Geometry: final body of the model. Coordinates: model frame, mm. Face numbers are marked on the shaded views. A direction names the side the tool comes from. Give positions to 0.01 mm unless a question says otherwise; leave off trailing zeros. Order: outer loops, then holes, each group sorted by start corner. A loop starts at its lowest first (then second) coordinate and runs counter-clockwise, first axis right, second up. Notation, with made-up numbers: (69.5, -38.75) - (107.5, -38.75) arc R23 cw to (107.5, 0.25) - close; hole circle Ø11 at (-10.5, 61.5). An arc over 180 degrees is marked (long way). Put each result on its own line as item: value. Start each with the question number.
1. Set-up query: the marked faces 4, 5, 6 and 7. Return all of +Z, -Z, +X, -X, +Y, -Y with unobstructed straight access to the full face (end or side cutting, diameter ignored); none if empty.
2. First-contact query: P1, Ø0.9, axis at x = 3, z = -3.5, coming from the +Y side; P2, Ø3.5, axis at x = -2, z = 17, coming from the -Y side; P3, Ø1, axis at x = 7, z = -1, coming from the +Y side. Flat tips, straight axial feed; report the tip coordinate or a pass-through.
3. Mould query, pull axis Z, two halves, no side actions, for the marked faces 1, 2 and 3. Classes: pulls with the +Z half, pulls with the -Z half, needs draft (parallel to the pull), parting line crosses it, or undercut.
4. Ray query, line 1 along Z through (x, y) = (-5.75, -13); line 2 along Z through (x, y) = (7.75, -20.5); line 3 along Z through (x, y) = (10.75, -16.5). Return the intervals inside material, ascending. Write a range as from..to.
5. Section B-B on x = 6.5. Count the separate pieces of the cut face and the enclosed holes in it, plus the area to 3 significant figures.
6. Section A-A on z = 17.5. Return the cut outline in (x, y).
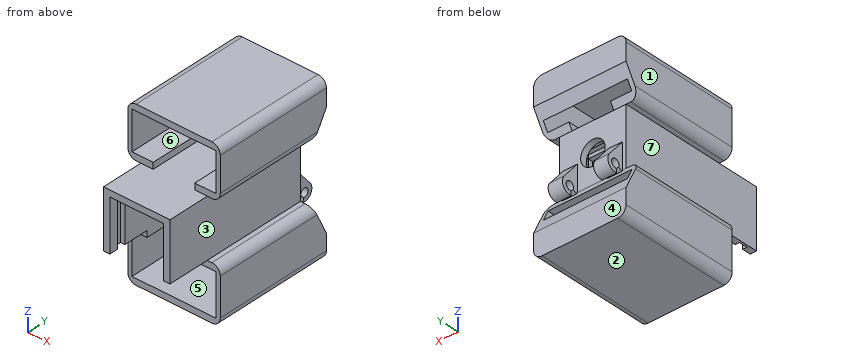
from build123d import *

# Parameters (mm, degrees)
SKETCH_1_W               = 12.8
SKETCH_1_H               = 10.8
EXTRUDE_1_DEPTH          = 1.5
CUT_EXTRUDE_1_REACH      = 13.721
SKETCH_2_R               = 2.9
SKETCH_3_W               = 12.8
SKETCH_3_H               = 1.5
EXTRUDE_2_DEPTH          = 35
SKETCH_6_W               = 12.8
SKETCH_6_H               = 1.5
CUT_EXTRUDE_2_DEPTH      = 10
EXTRUDE_4_DEPTH          = 15.8
CUT_EXTRUDE_3_DEPTH      = 38.580939349
CUT_EXTRUDE_3_DEPTH_BACK = 38.580939349
SKETCH_10_W              = 7.4
SKETCH_10_H              = 4
SKETCH_10_W_2            = 0.8
EXTRUDE_5_DEPTH          = 3.1
EXTRUDE_5_DEPTH_BACK     = 18.9
SKETCH_18_W              = 20
SKETCH_18_H              = 10
CUT_EXTRUDE_4_DEPTH      = 27
CUT_EXTRUDE_5_REACH      = 40.777
SKETCH_20_W              = 12.8
SKETCH_20_H              = 11.75
FILLET_3_R               = 2
SKETCH_21_W              = 12.8
SKETCH_21_H              = 33.5
EXTRUDE_6_DEPTH          = 0.8
SKETCH_22_W              = 12.8
SKETCH_22_H              = 10
CUT_EXTRUDE_6_DEPTH      = 0.8
SKETCH_23_W              = 12.8
SKETCH_23_H              = 2
CUT_EXTRUDE_7_DEPTH      = 0.8
SKETCH_25_W              = 12.8
SKETCH_25_H              = 2
CUT_EXTRUDE_8_DEPTH      = 0.8
SKETCH_26_W              = 12.8
SKETCH_26_H              = 2
CUT_EXTRUDE_9_DEPTH      = 0.8
SKETCH_27_W              = 12.8
SKETCH_27_H              = 2
CUT_EXTRUDE_10_DEPTH     = 0.8
SKETCH_28_W              = 10
SKETCH_28_H              = 2
CUT_EXTRUDE_11_DEPTH     = 0.3
SKETCH_29_W              = 10
SKETCH_29_H              = 2
CUT_EXTRUDE_12_DEPTH     = 0.3
SKETCH_30_W              = 22
SKETCH_30_H              = 28.5
EXTRUDE_7_DEPTH          = 12.2
SKETCH_32_W              = 20
SKETCH_32_H              = 9.2
CUT_EXTRUDE_13_DEPTH     = 27
CUT_EXTRUDE_14_DEPTH     = 46.551260858
SKETCH_34_W              = 9.9
SKETCH_34_H              = 1.5
CUT_EXTRUDE_15_DEPTH     = 39.481186787
FILLET_4_R               = 2
SKETCH_36_W              = 12.3
SKETCH_36_H              = 2
CUT_EXTRUDE_18_DEPTH     = 1
SKETCH_37_W              = 12.3
SKETCH_37_H              = 2
CUT_EXTRUDE_19_DEPTH     = 1


with BuildPart() as part:
    # 草图1 → 凸台-拉伸1 (new body)
    with BuildSketch(Plane(origin=(0, 0, 0), x_dir=(1, 0, 0), z_dir=(0, 1, 0))):
        with Locations((2.081833616, -2.548726655)):
            Rectangle(SKETCH_1_W, SKETCH_1_H)
    extrude(amount=EXTRUDE_1_DEPTH)

    # 草图2 → 切除-拉伸1 (cut, up to next)
    with BuildSketch(Plane(origin=(0, 1.5, 0), x_dir=(1, 0, 0), z_dir=(0, 1, 0)), mode=Mode.PRIVATE) as cut_extrude_1_sk1:
        with Locations(Location((2.081833616, -2.548726655, 0), (0, 0, 270))):
            Circle(SKETCH_2_R)
    cut_extrude_1_tool1 = extrude(cut_extrude_1_sk1.sketch, amount=-CUT_EXTRUDE_1_REACH, mode=Mode.PRIVATE) & part.part
    add(cut_extrude_1_tool1.solids().sort_by_distance((2.081834, 1.5, 2.548727))[0], mode=Mode.SUBTRACT)

    # 草图3 → 凸台-拉伸2 (add)
    with BuildSketch(Plane(origin=(0, 1.5, 0), x_dir=(1, 0, 0), z_dir=(0, 1, 0))):
        Polygon((-4.318166384, 4.351273345), (-5.818166384, 4.351273345), (-5.818166384, -9.448726655), (-4.318166384, -9.448726655), (-4.318166384, -7.948726655), (-4.318166384, 2.851273345), align=None)
        with Locations((2.081833616, 3.601273345)):
            Rectangle(SKETCH_3_W, SKETCH_3_H)
        Polygon((8.481833616, 4.351273345), (9.981833616, 4.351273345), (9.981833616, -9.448726655), (8.481833616, -9.448726655), (8.481833616, -7.948726655), (8.481833616, 2.851273345), align=None)
        with Locations((2.081833616, -8.698726655)):
            Rectangle(SKETCH_3_W, SKETCH_3_H)
    extrude(amount=-EXTRUDE_2_DEPTH)

    # 草图6 → 切除-拉伸2 (cut)
    with BuildSketch(Plane.XZ.offset(33.5)):
        with Locations((2.081833616, -3.601273345)):
            Rectangle(SKETCH_6_W, SKETCH_6_H)
    extrude(amount=-CUT_EXTRUDE_2_DEPTH, mode=Mode.SUBTRACT)

    # 草图9 → 凸台-拉伸4 (add)
    with BuildSketch(Plane(origin=(9.981833616, 0, 0), x_dir=(0, 0, -1), z_dir=(1, 0, 0))):
        with BuildLine():
            Line((4.294951619, 2.603813865), (4.738629893, 1.70762773))
            ThreePointArc((4.738629893, 1.70762773), (4.306935204, 1.552598585), (3.851273345, 1.5))
            Line((3.851273345, 1.5), (-1.771682581, 1.5))
            Line((-1.771682581, 1.5), (2.59831793, 5.058878677))
            ThreePointArc((2.59831793, 5.058878677), (4.892528233, 5.207567937), (5.810847908, 3.099915598))
            Line((5.810847908, 3.099915598), (4.830532954, 3.297390482))
            ThreePointArc((4.830532954, 3.297390482), (3.059787283, 4.111187217), (4.294951619, 2.603813865))
        make_face()
    extrude(amount=-EXTRUDE_4_DEPTH)

    # 草图10 → 切除-拉伸3 (cut, two sides: drawn at the far end of the back side and taken through both)
    with BuildSketch(Plane(origin=(0, 0, -4.351273345), x_dir=(-1, 0, 0), z_dir=(0, 0, -1)).offset(-CUT_EXTRUDE_3_DEPTH_BACK)):
        with Locations((-2.081833616, 3.5)):
            Rectangle(SKETCH_10_W, SKETCH_10_H)
        with Locations((5.418166384, 3.5)):
            Rectangle(SKETCH_10_W_2, SKETCH_10_H)
        with Locations((-9.581833616, 3.5)):
            Rectangle(SKETCH_10_W_2, SKETCH_10_H)
    extrude(amount=CUT_EXTRUDE_3_DEPTH + CUT_EXTRUDE_3_DEPTH_BACK, mode=Mode.SUBTRACT)

    # 草图17 → 凸台-拉伸5 (add, two sides: drawn at the far end of the back side and taken through both)
    with BuildSketch(Plane.ZY.offset(5.818166384).offset(-EXTRUDE_5_DEPTH_BACK)):
        Polygon((-4.351273345, -23.5), (-17.351273345, -23.5), (-17.351273345, 5), (-11.601273345, 5), (-4.351273345, 1.5), align=None)
    extrude(amount=EXTRUDE_5_DEPTH + EXTRUDE_5_DEPTH_BACK)

    # 草图18 → 切除-拉伸4 (cut)
    with BuildSketch(Plane.XZ.offset(23.5)):
        with Locations((2.081833616, -10.851273345)):
            Rectangle(SKETCH_18_W, SKETCH_18_H)
    extrude(amount=-CUT_EXTRUDE_4_DEPTH, mode=Mode.SUBTRACT)

    # 草图20 → 切除-拉伸5 (cut, up to next)
    with BuildSketch(Plane.XY.offset(-2.851273345), mode=Mode.PRIVATE) as cut_extrude_5_sk1:
        with Locations((2.081833616, -17.625)):
            Rectangle(SKETCH_20_W, SKETCH_20_H)
    cut_extrude_5_tool1 = extrude(cut_extrude_5_sk1.sketch, amount=-CUT_EXTRUDE_5_REACH, mode=Mode.PRIVATE) & part.part
    add(cut_extrude_5_tool1.solids().sort_by_distance((2.081834, -17.625, -2.851273))[0], mode=Mode.SUBTRACT)

    # 圆角3
    fillet_3_edges = [part.edges().sort_by_distance(p)[0] for p in [
        (13.081833616, -11, -4.351273345),
        (13.081833616, -9.25, -17.351273345),
        (-8.918166384, -11, -4.351273345),
        (-8.918166384, -9.25, -17.351273345),
    ]]
    fillet(fillet_3_edges, radius=FILLET_3_R)

    # 草图21 → 凸台-拉伸6 (add)
    with BuildSketch(Plane(origin=(0, 0, 7.948726655), x_dir=(-1, 0, 0), z_dir=(0, 0, -1))):
        with Locations((-2.081833616, -16.75)):
            Rectangle(SKETCH_21_W, SKETCH_21_H)
    extrude(amount=EXTRUDE_6_DEPTH)

    # 草图22 → 切除-拉伸6 (cut)
    with BuildSketch(Plane(origin=(0, 0, 7.148726655), x_dir=(-1, 0, 0), z_dir=(0, 0, -1))):
        with Locations((-2.081833616, -28.5)):
            Rectangle(SKETCH_22_W, SKETCH_22_H)
    extrude(amount=-CUT_EXTRUDE_6_DEPTH, mode=Mode.SUBTRACT)

    # 草图23 → 切除-拉伸7 (cut)
    with BuildSketch(Plane(origin=(0, 0, 7.148726655), x_dir=(-1, 0, 0), z_dir=(0, 0, -1))):
        with Locations((-2.081833616, -3.5)):
            Rectangle(SKETCH_23_W, SKETCH_23_H)
    extrude(amount=-CUT_EXTRUDE_7_DEPTH, mode=Mode.SUBTRACT)

    # 草图25 → 切除-拉伸8 (cut)
    with BuildSketch(Plane.XY.offset(-2.851273345)):
        with Locations((2.081833616, -3.5)):
            Rectangle(SKETCH_25_W, SKETCH_25_H)
    extrude(amount=-CUT_EXTRUDE_8_DEPTH, mode=Mode.SUBTRACT)

    # 草图26 → 切除-拉伸9 (cut)
    with BuildSketch(Plane(origin=(0, 0, 7.148726655), x_dir=(-1, 0, 0), z_dir=(0, 0, -1))):
        with Locations((-2.081833616, -6.6)):
            Rectangle(SKETCH_26_W, SKETCH_26_H)
    extrude(amount=-CUT_EXTRUDE_9_DEPTH, mode=Mode.SUBTRACT)

    # 草图27 → 切除-拉伸10 (cut)
    with BuildSketch(Plane.XY.offset(-2.851273345)):
        with Locations((2.081833616, -6.6)):
            Rectangle(SKETCH_27_W, SKETCH_27_H)
    extrude(amount=-CUT_EXTRUDE_10_DEPTH, mode=Mode.SUBTRACT)

    # 草图28 → 切除-拉伸11 (cut)
    with BuildSketch(Plane(origin=(-4.318166384, 0, 0), x_dir=(0, 0, -1), z_dir=(1, 0, 0))):
        with Locations((-2.148726655, -6.6)):
            Rectangle(SKETCH_28_W, SKETCH_28_H)
        with Locations((-2.148726655, -3.5)):
            Rectangle(SKETCH_28_W, SKETCH_28_H)
    extrude(amount=-CUT_EXTRUDE_11_DEPTH, mode=Mode.SUBTRACT)

    # 草图29 → 切除-拉伸12 (cut)
    with BuildSketch(Plane.ZY.offset(-8.481833616)):
        with Locations((2.148726655, -3.5)):
            Rectangle(SKETCH_29_W, SKETCH_29_H)
        with Locations((2.148726655, -6.6)):
            Rectangle(SKETCH_29_W, SKETCH_29_H)
    extrude(amount=-CUT_EXTRUDE_12_DEPTH, mode=Mode.SUBTRACT)

    # 草图30 → 凸台-拉伸7 (add)
    with BuildSketch(Plane.XY.offset(9.448726655)):
        with Locations((2.081833616, -9.25)):
            Rectangle(SKETCH_30_W, SKETCH_30_H)
    extrude(amount=EXTRUDE_7_DEPTH)

    # 草图32 → 切除-拉伸13 (cut)
    with BuildSketch(Plane.XZ.offset(23.5)):
        with Locations((2.081833616, 15.548726655)):
            Rectangle(SKETCH_32_W, SKETCH_32_H)
    extrude(amount=-CUT_EXTRUDE_13_DEPTH, mode=Mode.SUBTRACT)

    # 草图33 → 切除-拉伸14 (cut, through all)
    with BuildSketch(Plane(origin=(13.081833616, 0, 0), x_dir=(0, 0, -1), z_dir=(1, 0, 0))):
        Polygon((-15.548726655, 5), (-9.448726655, 1.5), (-9.448726655, 5), align=None)
    extrude(amount=-CUT_EXTRUDE_14_DEPTH, mode=Mode.SUBTRACT)

    # 草图34 → 切除-拉伸15 (cut, through all)
    with BuildSketch(Plane.XZ.offset(23.5)):
        with Locations((2.065568836, 10.198726655)):
            Rectangle(SKETCH_34_W, SKETCH_34_H)
    extrude(amount=-CUT_EXTRUDE_15_DEPTH, mode=Mode.SUBTRACT)

    # 圆角4
    fillet_4_edges = [part.edges().sort_by_distance(p)[0] for p in [
        (13.081833616, -11, 9.448726655),
        (-8.918166384, -9.25, 21.648726655),
        (13.081833616, -9.25, 21.648726655),
        (-8.918166384, -11, 9.448726655),
    ]]
    fillet(fillet_4_edges, radius=FILLET_4_R)

    # 草图36 → 切除-拉伸18 (cut)
    with BuildSketch(Plane(origin=(-4.318166384, 0, 0), x_dir=(0, 0, -1), z_dir=(1, 0, 0))):
        with Locations((-1.798726655, -30.5)):
            Rectangle(SKETCH_36_W, SKETCH_36_H)
    extrude(amount=-CUT_EXTRUDE_18_DEPTH, mode=Mode.SUBTRACT)

    # 草图37 → 切除-拉伸19 (cut)
    with BuildSketch(Plane.ZY.offset(-8.481833616)):
        with Locations((1.798726655, -30.5)):
            Rectangle(SKETCH_37_W, SKETCH_37_H)
    extrude(amount=-CUT_EXTRUDE_19_DEPTH, mode=Mode.SUBTRACT)


solid = part.part
Resolved:
1. face 4: -Z, +X, -X, +Y
1. face 5: -Y
1. face 6: +Y, -Y
1. face 7: -X, +Y, -Y
2. P1: y = 1.5
2. P2: y = 3.5
2. P3: y = 4.16
3. face 1: needs draft
3. face 2: pulls with the -Z half
3. face 3: undercut
4. line 1: -17.35..-15.85, -5.85..10.95, 20.15..21.65
4. line 2: -17.35..-15.85, 7.15..10.95, 20.15..21.65
4. line 3: -17.35..-15.85, -5.85..-4.35, 9.45..10.95, 20.15..21.65
5. separate pieces: 3
5. enclosed holes: 0
5. area: 239 mm^2
6. outline: (-8.92, -23.5) - (-7.92, -23.5) - (-7.92, 3.5) - (12.08, 3.5) - (12.08, -23.5) - (13.08, -23.5) - (13.08, 5) - (-8.92, 5) - close
